```python
from build123d import *

# Parameters (mm, degrees)
ESTRUSIONE_ESTRUSIONE1_START     = -4
ESTRUSIONE_ESTRUSIONE1_OUTLINE_R = 1.75
ESTRUSIONE_ESTRUSIONE1_DEPTH     = 8
SCHIZZO2_W                       = 5
SCHIZZO2_H                       = 30
TAGLIO_ESTRUSIONE1_DEPTH         = 15


# Read off the part's stored shape, not the designer's step: Estrusione-Estrusione1
with BuildPart() as part:
    # Estrusione-Estrusione1 outline → Estrusione-Estrusione1 (new body)
    with BuildSketch(Plane.XY.offset(ESTRUSIONE_ESTRUSIONE1_START)):
        with BuildLine():
            Line((-25.284658439, 35.888314388), (-18.737560358, 34.376797697))
            Line((-18.737560358, 34.376797697), (-18.90016625, 40.460566904))
            Line((-18.90016625, 40.460566904), (-19.768803662, 40.460566904))
            ThreePointArc((-19.768803662, 40.460566904), (-22.136039573, 52.710253398), (-19.768803662, 64.959939892))
            Line((-19.768803662, 64.959939892), (-19.554981097, 64.959939892))
            Line((-19.554981097, 64.959939892), (-19.767739779, 72.920135539))
            Line((-19.767739779, 72.920135539), (-22.627052267, 71.534084223))
            Line((-22.627052267, 71.534084223), (-29.102672814, 57.04304198))
            Line((-29.102672814, 57.04304198), (-38.990570649, 26.611221593))
            ThreePointArc((-38.990570649, 26.611221593), (-36.850363143, 21.914964836), (-32.358508436, 24.456333953))
            Line((-32.358508436, 24.456333953), (-29.400684937, 33.559578642))
            ThreePointArc((-29.400684937, 33.559578642), (-27.79546959, 35.524264097), (-25.284658439, 35.888314388))
        make_face()
        with Locations((-35.768803662, 25.243662643)):
            Circle(ESTRUSIONE_ESTRUSIONE1_OUTLINE_R, mode=Mode.SUBTRACT)
        with Locations((-30.824531752, 40.460566904)):
            Circle(ESTRUSIONE_ESTRUSIONE1_OUTLINE_R, mode=Mode.SUBTRACT)
    extrude(amount=ESTRUSIONE_ESTRUSIONE1_DEPTH)

    # Schizzo2 → Taglio-Estrusione1 (cut, symmetric)
    with BuildSketch(Plane(origin=(-39.772113155, 12.922742925, 0), x_dir=(0, 0, 1), z_dir=(-0.9510565162951534, 0.3090169943749484, 0))):
        with Locations((0, 17.257936303)):
            Rectangle(SCHIZZO2_W, SCHIZZO2_H)
    extrude(amount=TAGLIO_ESTRUSIONE1_DEPTH, both=True, mode=Mode.SUBTRACT)


solid = part.part
```
Here's how the part is built. I have some questions about the finished solid (model axes, mm). A direction names the side the tool comes from. Give positions to 0.01 mm unless a question says otherwise; leave off trailing zeros. Order: outer loops, then holes, each group sorted by start corner. A loop starts at its lowest first (then second) coordinate and runs counter-clockwise, first axis right, second up. Notation, with made-up numbers: (10.5, -5) - (37.5, -5) arc R18 ccw to (37.5, 6) - close; hole circle Ø4 at (56.5, 40). An arc over 180 degrees is marked (long way). Answer as a JSON object with one key per item and string values. Group by question number.
Item 1: If we section it at C-C on z = -1: Please give me the cut outline in (x, y), and give its area (3 significant figures).
Item 2: If we section it at D-D on y = 37.5: Please give me the cut outline in (x, z).
Item 3: If we mould it in two halves opening along X, with no side actions, what happens to faces 1 (the flat face through (-22.057, 35.143, -3.26)), 2 (the flat face through (-30.9, 28.94, -3.26)), 3 (the flat face through (-26.1, 42.4, 0))? For each: pulls with the +X half, pulls with the -X half, needs draft (parallel to the pull), parting line crosses it, or undercut.
Item 4: Which directions (+Z, -Z, +X, -X, +Y, -Y) give clear straight access to the entire face, cutting with the end or side of a thin tool? Please do faces 4 (the cylindrical face through (-27.827, 35.506, -3.26)), 5 (the flat face through (-19.3, 40.461, -0.1)), 6 (the flat face through (-30, 34, 2.5)).
Item 5: If we section it at A-A on x = -30.25: Please give me the cut outline in (y, z), and give its area (3 significant figures).
Item 6: If we section it at B-B on x = -20.75: Please give me the cut outline in (y, z).
Item 7: For P1, Ø3, axis at x = -35.77, y = 25.24, coming from the +Z side; P2, Ø10.5, axis at x = -27.5, y = 32.5, coming from the +Z side; P3, Ø1, axis at x = -21, z = -1, coming from the -Y side; P4, Ø1.5, axis at x = -32, z = -1.5, coming from the -Y side, each with a flat end and sliding along its axis, tell me the tip position at first contact or that it passes through.
Item 8: Please list where these lines run through material, in increasing order: probe 1 along Z at (x, y) = (-24.5, 37); probe 2 along Y at (x, z) = (-28.5, -2.75); probe 3 along X at (y, z) = (52, 2.25).
Result set:
{
 "1": {"outline": "(-33.12, 44.68) - (-18.89, 40.06) - (-18.9, 40.46) - (-19.77, 40.46) arc R32.88 cw to (-19.77, 64.96) - (-19.55, 64.96) - (-19.77, 72.92) - (-22.63, 71.53) - (-29.1, 57.04) - close", "area": "222 mm²"},
 "2": {"outline": "(-35.45, -4) - (-18.82, -4) - (-18.82, -2.5) - (-35.45, -2.5) - close; (-35.45, 2.5) - (-18.82, 2.5) - (-18.82, 4) - (-35.45, 4) - close"},
 "3": {"face 1": "undercut", "face 2": "pulls with the +X half", "face 3": "pulls with the -X half"},
 "4": {"face 4": "+Z, -Z, -Y", "face 5": "+Z, -Z, +X", "face 6": "-X, -Y"},
 "5": {"outline": "(30.95, -4) - (38.81, -4) - (38.81, -2.5) - (30.95, -2.5) - close; (30.95, 2.5) - (38.81, 2.5) - (38.81, 4) - (30.95, 4) - close; (42.11, -4) - (53.51, -4) - (53.51, 4) - (42.11, 4) - (42.11, 2.5) - (43.75, 2.5) - (43.75, -2.5) - (42.11, -2.5) - close", "area": "107 mm²"},
 "6": {"outline": "(34.84, -4) - (43.26, -4) - (43.26, 4) - (34.84, 4) - (34.84, 2.5) - (40.66, 2.5) - (40.66, -2.5) - (34.84, -2.5) - close; (62.16, -4) - (72.44, -4) - (72.44, 4) - (62.16, 4) - close"},
 "7": {"P1": "through", "P2": "z = 4", "P3": "y = 40.58", "P4": "y = 44.07"},
 "8": {"probe 1": "-4 to -2.5, 2.5 to 4", "probe 2": "35 to 58.39", "probe 3": "-30.74 to -22.13"}
}
